Here's how the part is built. I have some questions about the finished solid (model axes, mm). A direction names the side the tool comes from. Round coordinates to 2 decimals unless told otherwise and drop trailing zeros. Order: outer loops, then holes, each group sorted by start corner. A loop starts at its lowest first (then second) coordinate and runs counter-clockwise, first axis right, second up. Notation, with made-up numbers: (67, 74) -> (113, 74) arc R31 cw to (113, 110) -> close; hole circle Ø5 at (-31, 4). An arc over 180 degrees is marked (long way). Use a Markdown table: item, result. Add a question column.
from build123d import *

# Parameters (mm, degrees)
SKETCH1_R           = 12.5
BOSS_EXTRUDE1_DEPTH = 30
SKETCH2_R           = 10
BOSS_EXTRUDE2_DEPTH = 11
SKETCH3_R           = 4.1
CUT_EXTRUDE1_DEPTH  = 318.401165719


with BuildPart() as part:
    # Sketch1 → Boss-Extrude1 (new body)
    with BuildSketch(Plane.XY):
        with Locations((25, -300)):
            Circle(SKETCH1_R)
    extrude(amount=-BOSS_EXTRUDE1_DEPTH)

    # Sketch2 → Boss-Extrude2 (add)
    with BuildSketch(Plane(origin=(0, 0, -30), x_dir=(-1, 0, 0), z_dir=(0, 0, -1))):
        with Locations(Location((-25, -300, 0), (0, 0, 180))):
            Circle(SKETCH2_R)
    extrude(amount=BOSS_EXTRUDE2_DEPTH)

    # Sketch3 → Cut-Extrude1 (cut, through all)
    with BuildSketch(Plane(origin=(0, 0, -41), x_dir=(-1, 0, 0), z_dir=(0, 0, -1))):
        with Locations((-25, -300)):
            Circle(SKETCH3_R)
    extrude(amount=-CUT_EXTRUDE1_DEPTH, mode=Mode.SUBTRACT)


solid = part.part
(1) If we mould it in two halves opening along Z, with no side actions, what happens to faces 3 (the flat face through (25, -305, 0)), 4 (the cylindrical face through (30.77, -311.09, -14.79)), 5 (the flat face through (24.9, -289.8, -30))? For each: pulls with the +Z half, pulls with the -Z half, needs draft (parallel to the pull), parting line crosses it, or undercut.
(2) I want a section at D-D on x = 30.75. List the corners of the cut face in (y, z) for me.
(3) Please list where these lines run through material, in increasing order: probe 1 along Y at (x, z) = (25, -28); probe 2 along Y at (x, z) = (25, -34); probe 3 along Z at (x, y) = (35, -293.75). Write a range as from..to.
(4) I want a section at B-B on x = 25. List the corners of the cut face in (y, z) for me.
(5) I want a section at A-A on y = -300. List the corners of the cut face in (x, z) for me.
(6) I want a section at C-C on z = -35.5. List the corners of the cut face in (x, y) for me, and give its area (3 significant figures).
(7) I'm going to push flat-ended pins straight in: P1, Ø8, axis at y = -294.5, z = -35, coming from the +X side; P2, Ø5, axis at y = -293.5, z = -26.5, coming from the -X side; P3, Ø6.5, axis at x = 25, y = -300, coming from the +Z side; P4, Ø2, axis at y = -306, z = -19, coming from the -X side. Where does each tip first touch, or does it pass through?
(8) On a 3-axis mill with a long thin cutter (end or side, diameter ignored), from which of +Z, -Z, +X, -X, +Y, -Y can I reach the whole of each face in a straight line? I mean faces 1 (the flat face through (29.3, -300.1, -41)), 2 (the cylindrical face through (29.614, -291.128, -35.423)). Say none if no direction works.
Output:
| question | item | result |
|---|---|---|
| 1 | face 3 | pulls with the +Z half |
| 1 | face 4 | needs draft |
| 1 | face 5 | pulls with the -Z half |
| 2 | outline | (-311.1, -30) -> (-308.18, -30) -> (-308.18, -41) -> (-291.82, -41) -> (-291.82, -30) -> (-288.9, -30) -> (-288.9, 0) -> (-311.1, 0) -> close |
| 3 | probe 1 | -312.5..-304.1, -295.9..-287.5 |
| 3 | probe 2 | -310..-304.1, -295.9..-290 |
| 3 | probe 3 | -30..0 |
| 4 | outline | (-312.5, -30) -> (-310, -30) -> (-310, -41) -> (-304.1, -41) -> (-304.1, 0) -> (-312.5, 0) -> close; (-295.9, -41) -> (-290, -41) -> (-290, -30) -> (-287.5, -30) -> (-287.5, 0) -> (-295.9, 0) -> close |
| 5 | outline | (12.5, -30) -> (15, -30) -> (15, -41) -> (20.9, -41) -> (20.9, 0) -> (12.5, 0) -> close; (29.1, -41) -> (35, -41) -> (35, -30) -> (37.5, -30) -> (37.5, 0) -> (29.1, 0) -> close |
| 6 | outline | circle Ø20 at (25, -300); hole circle Ø8.2 at (25, -300) |
| 6 | area | 261 mm² |
| 7 | P1 | x = 34.89 |
| 7 | P2 | x = 13.16 |
| 7 | P3 | through |
| 7 | P4 | x = 13.54 |
| 8 | face 1 | -Z, +X, -X, +Y, -Y |
| 8 | face 2 | -Z |
